Work out the finished part from the listing and answer in its coordinate system (mm). A direction names the side the tool comes from. Give positions to 0.01 mm unless a question says otherwise; leave off trailing zeros. Write each loop counter-clockwise with the first axis right and the second up, starting at its lowest first coordinate (ties: lowest second). Pieces come first, ordered by that corner, then holes. Notation, with made-up numbers: (-27, 72.5) -> (28, 72.5) arc R12 ccw to (28, 80.5) -> close; hole circle Ø5 at (35, 37). An arc over 180 degrees is marked (long way). Write item = value, one per line. Start each with the question number.
Autodesk Inventor part; units mm, degrees
ref_plane "YZ Plane" through (0, 0, 0) normal (1, 0, 0) x (0, 1, 0)
ref_plane "XZ Plane" through (0, 0, 0) normal (0, 1, 0) x (-1, 0, 0)
ref_plane "XY Plane" through (0, 0, 0) normal (0, 0, 1) x (1, 0, 0)
sketch "Sketch1" plane through (0, 0, 0) normal (0, 0, 1) x (1, 0, 0)
  line L0 (-4.8133, 6.477) -> (4.8133, 6.477)
  line L1 (4.8133, 6.477) -> (4.8133, -6.477)
  line L2 (4.8133, -6.477) -> (-4.8133, -6.477)
  line L3 (-4.8133, -6.477) -> (-4.8133, 6.477)
  line L4 (-4.8133, 6.477) -> (4.8133, -6.477) construction
  line L5 (4.8133, 6.477) -> (-4.8133, -6.477) construction
  point P0 (0, 0)
extrude "Extrusion1" add sketch "Sketch1" along normal blind 7.874
sketch "Sketch2" plane through (0, 0, 0) normal (0, 0, -1) x (-1, 0, 0)
  line L0 (-1.0414, 4.7498) -> (1.0414, 4.7498)
  line L1 (1.0414, 4.7498) -> (1.0414, 3.9878)
  line L2 (1.0414, 3.9878) -> (-1.0414, 3.9878)
  line L3 (-1.0414, 3.9878) -> (-1.0414, 4.7498)
  line L4 (-1.0414, 4.7498) -> (1.0414, 3.9878) construction
  line L5 (1.0414, 4.7498) -> (-1.0414, 3.9878) construction
  line L6 (4.8133, 6.477) -> (-4.8133, 6.477)
  point P0 (0, 0)
  point P1 (0, 4.3688)
  dimension "d7" = 2.0828
  dimension "d8" = 0.762
  dimension "d28" = 1.7272
extrude "Extrusion2" add sketch "Sketch2" along normal blind 3.9878
sketch "Sketch3" plane through (0, 0, 0) normal (0, 0, -1) x (-1, 0, 0)
  line L0 (-1.0414, 0.381) -> (1.0414, 0.381)
  line L1 (1.0414, 0.381) -> (1.0414, -0.381)
  line L2 (1.0414, -0.381) -> (-1.0414, -0.381)
  line L3 (-1.0414, -0.381) -> (-1.0414, 0.381)
  line L4 (-1.0414, 0.381) -> (1.0414, -0.381) construction
  line L5 (1.0414, 0.381) -> (-1.0414, -0.381) construction
  line L6 (-1.0414, 3.9878) -> (1.0414, 3.9878)
  line L7 (4.8133, 6.477) -> (-4.8133, 6.477)
  line L8 (1.0414, 4.7498) -> (-1.0414, 4.7498)
  point P0 (0, 0)
  point P1 (0, 0)
  dimension "d13" = 2.0828
  dimension "d15" = 0.762
  dimension "d16" = 3.6068
  dimension "d18" = 1.7272
extrude "Extrusion3" add sketch "Sketch3" along normal blind 3.9878
sketch "Sketch4" plane through (0, 0, 0) normal (0, 0, -1) x (-1, 0, 0)
  line L0 (-1.0414, -3.9878) -> (1.0414, -3.9878)
  line L1 (1.0414, -3.9878) -> (1.0414, -4.7498)
  line L2 (1.0414, -4.7498) -> (-1.0414, -4.7498)
  line L3 (-1.0414, -4.7498) -> (-1.0414, -3.9878)
  line L4 (-1.0414, -3.9878) -> (1.0414, -4.7498) construction
  line L5 (1.0414, -3.9878) -> (-1.0414, -4.7498) construction
  line L6 (-1.0414, -0.381) -> (1.0414, -0.381)
  line L7 (-4.8133, -6.477) -> (4.8133, -6.477)
  point P0 (0, 0)
  point P1 (0, -4.3688)
  dimension "d24" = 0.762
  dimension "d25" = 3.6068
  dimension "d27" = 2.0828
extrude "Extrusion4" add sketch "Sketch4" along normal blind 3.9878
sketch "Sketch5" plane through (0, 0, 7.874) normal (0, 0, 1) x (1, 0, 0)
  circle A0 centre (0, 0) radius 2.8448
  dimension "d31" = 5.6896
extrude "Extrusion5" add sketch "Sketch5" along normal blind 8.8646
sketch "Sketch6" plane through (0, 0, 16.7386) normal (0, 0, 1) x (1, 0, 0)
  circle A0 centre (0, 0) radius 1.5367
  dimension "d34" = 3.0734
extrude "Extrusion6" add sketch "Sketch6" along normal blind 9.3726
properties part number "Mini toggle switch"
(1) A cutting plane is placed at A-A, the plane z = -2. Write down the section's boundary in (x, y).
(2) Determine the mould class of faces 1 (the flat face through (1.2, -1.2, 16.739)), 2 (the cylindrical face through (-0.617, 2.777, 12.244)), 3 (the flat face through (0, 3.988, -2)) for opening direction Y: pulls with the +Y half, pulls with the -Y half, needs draft (parallel to the pull), parting line crosses it, or undercut.
(3) A cutting plane is placed at C-C, the plane x = 0. Write down the section's boundary in (y, z).
(4) For faces 4 (the flat face through (0, 3, 7.874)), 5 (the flat face through (0, 4.75, -2)), 6 (the flat face through (0, -0.381, -2)), determine the directions among +Z, -Z, +X, -X, +Y, -Y from which every point of the face is accessible in a straight line to the end or side of a thin tool.
(5) Find the intervals of material crossed by line 1 along Z through (x, y) = (-1, 5.5); line 2 along Z through (x, y) = (-2, -1); line 3 along X through (y, z) = (0.75, 10.5), in increasing order.
(6) A cutting plane is placed at D-D, the plane z = 15.5. Write down the section's boundary in (x, y), then the cut area to 3 significant figures.
(7) Each of these flat-tipped pins is pushed along its axis until it touches: pin 1 (0.8 mm diameter, centred on y = 0, z = -3, fed in from +X); pin 2 (2 mm diameter, centred on x = -2.5, y = 4.5, fed in from -Z); pin 3 (0.6 mm diameter, centred on y = -4.5, z = -1, fed in from -X); pin 4 (2 mm diameter, centred on x = -3.5, z = 20.5, fed in from -Y). Where does it stop, or does it pass through?
(8) A cutting plane is placed at B-B, the plane y = 0. Write down the section's boundary in (x, z).
Results list:
q1.outline = (-1.04, -4.75) -> (1.04, -4.75) -> (1.04, -3.99) -> (-1.04, -3.99) -> close; (-1.04, -0.38) -> (1.04, -0.38) -> (1.04, 0.38) -> (-1.04, 0.38) -> close; (-1.04, 3.99) -> (1.04, 3.99) -> (1.04, 4.75) -> (-1.04, 4.75) -> close
q2.face_1 = needs draft
q2.face_2 = parting line crosses it
q2.face_3 = undercut
q3.outline = (-6.48, 0) -> (-4.75, 0) -> (-4.75, -3.99) -> (-3.99, -3.99) -> (-3.99, 0) -> (-0.38, 0) -> (-0.38, -3.99) -> (0.38, -3.99) -> (0.38, 0) -> (3.99, 0) -> (3.99, -3.99) -> (4.75, -3.99) -> (4.75, 0) -> (6.48, 0) -> (6.48, 7.87) -> (2.84, 7.87) -> (2.84, 16.74) -> (1.54, 16.74) -> (1.54, 26.11) -> (-1.54, 26.11) -> (-1.54, 16.74) -> (-2.84, 16.74) -> (-2.84, 7.87) -> (-6.48, 7.87) -> close
q4.face_4 = +Z
q4.face_5 = -Z, +X, -X, +Y
q4.face_6 = -Z, +X, -X
q5.line_1 = 0 to 7.87
q5.line_2 = 0 to 16.74
q5.line_3 = -2.74 to 2.74
q6.outline = circle Ø5.69 at (0, 0)
q6.area = 25.4 mm²
q7.pin_1 = 1.04
q7.pin_2 = 0
q7.pin_3 = -1.04
q7.pin_4 = through
q8.outline = (-4.81, 0) -> (-1.04, 0) -> (-1.04, -3.99) -> (1.04, -3.99) -> (1.04, 0) -> (4.81, 0) -> (4.81, 7.87) -> (2.84, 7.87) -> (2.84, 16.74) -> (1.54, 16.74) -> (1.54, 26.11) -> (-1.54, 26.11) -> (-1.54, 16.74) -> (-2.84, 16.74) -> (-2.84, 7.87) -> (-4.81, 7.87) -> close
